Build history of the part. All positions in model axes, mm. Round coordinates to 2 decimals unless told otherwise and drop trailing zeros. Loops run counter-clockwise (first coordinate to the right, second up) from the corner with the lowest first, then second, coordinate; pieces in that order, holes last. Notation, with made-up numbers: (58.5, -1.75) - (77.5, -1.75) arc R13 ccw to (77.5, 7.25) - close; hole circle Ø4 at (79, 27.25). An arc over 180 degrees is marked (long way). Use a Markdown table: item, result.
from build123d import *

# Parameters (mm, degrees)
EXTRUDE_1_DEPTH        = 400
SKETCH_2_R             = 3
SKETCH_2_R_2           = 1.75
CUT_EXTRUDE_1_DEPTH    = 4.5
SKETCH_2_2_R           = 1.75
CUT_EXTRUDE_2_DEPTH    = 9
PATTERN_LINEAR_1_COUNT = 14
PATTERN_LINEAR_1_PITCH = 25
CROQUIS1_R             = 1.75
CORTAR_EXTRUIR1_DEPTH  = 8


with BuildPart() as part:
    # Эскиз1 → Бобышка-Вытянуть1 (new body)
    with BuildSketch(Plane.XY):
        with BuildLine():
            Line((-6, 3.7), (-5.7, 4))
            Line((-5.7, 4), (5.7, 4))
            Line((5.7, 4), (6, 3.7))
            Line((6, 3.7), (6, 2.451013544))
            ThreePointArc((6, 2.451013544), (5.597935912, 2.202976267), (5.354599002, 1.798050138))
            Line((5.354599002, 1.798050138), (4.643514056, 1.798050138))
            Line((4.643514056, 1.798050138), (4.643514056, 1.201949862))
            Line((4.643514056, 1.201949862), (5.354599002, 1.201949862))
            ThreePointArc((5.354599002, 1.201949862), (5.597935912, 0.797023733), (6, 0.548986456))
            Line((6, 0.548986456), (6, -3.7))
            Line((6, -3.7), (5.7, -4))
            Line((5.7, -4), (-5.7, -4))
            Line((-5.7, -4), (-6, -3.7))
            Line((-6, -3.7), (-6, 0.548986456))
            ThreePointArc((-6, 0.548986456), (-5.597935912, 0.797023733), (-5.354599002, 1.201949862))
            Line((-5.354599002, 1.201949862), (-4.643514056, 1.201949862))
            Line((-4.643514056, 1.201949862), (-4.643514056, 1.798050138))
            Line((-4.643514056, 1.798050138), (-5.354599002, 1.798050138))
            ThreePointArc((-5.354599002, 1.798050138), (-5.597935912, 2.202976267), (-6, 2.451013544))
            Line((-6, 2.451013544), (-6, 3.7))
        make_face()
    extrude(amount=EXTRUDE_1_DEPTH)

    # Эскиз2 → Вырез-Вытянуть1 (cut)
    with BuildSketch(Plane(origin=(0, 4, 0), x_dir=(1, 0, 0), z_dir=(0, 1, 0))):
        with Locations((0, -12)):
            Circle(SKETCH_2_R)
        with Locations((0, -12)):
            Circle(SKETCH_2_R_2, mode=Mode.SUBTRACT)
    cut_extrude_1 = extrude(amount=-CUT_EXTRUDE_1_DEPTH, mode=Mode.SUBTRACT)

    # Эскиз2<2> → Вырез-Вытянуть2 (cut, through all)
    with BuildSketch(Plane(origin=(0, 4, 0), x_dir=(1, 0, 0), z_dir=(0, 1, 0))):
        with Locations((0, -12)):
            Circle(SKETCH_2_2_R)
    cut_extrude_2 = extrude(amount=-CUT_EXTRUDE_2_DEPTH, mode=Mode.SUBTRACT)

    # Линейный массив1: Вырез-Вытянуть1, Вырез-Вытянуть2 ×14
    with Locations(*[(0, 0, i * PATTERN_LINEAR_1_PITCH) for i in range(1, PATTERN_LINEAR_1_COUNT)]):
        add(cut_extrude_1, mode=Mode.SUBTRACT)
        add(cut_extrude_2, mode=Mode.SUBTRACT)

    # Croquis1 → Cortar-Extruir1 (cut)
    with BuildSketch(Plane(origin=(0, 4, 0), x_dir=(1, 0, 0), z_dir=(0, 1, 0))):
        with Locations((0, -388)):
            Circle(CROQUIS1_R)
        with Locations((0, -363)):
            Circle(CROQUIS1_R)
    extrude(amount=-CORTAR_EXTRUIR1_DEPTH, mode=Mode.SUBTRACT)


solid = part.part
Q1. Drop flat-ended pins along their axis: pin 1 (5.5 mm diameter, centred on x = 0, z = 312, fed in from +Y); pin 2 (3 mm diameter, centred on x = 0, z = 37, fed in from +Y). Give the stop position or say it passes through.
Results found:
| item | result |
|---|---|
| pin 1 | stops at y = -0.5 |
| pin 2 | passes through |
Q2. Probe line 1 (Y direction, x = -5.25, z = 59.5); line 2 (X direction, y = -0.25, z = 137); line 3 (X direction, y = 1.75, z = 212). List the from-to ranges inside material, lowest first.
Results found:
| item | result |
|---|---|
| line 1 | y = -4 to 1.2, 1.8 to 4 |
| line 2 | x = -6 to -3, 3 to 6 |
| line 3 | x = -4.64 to -3, 3 to 4.64 |
Q3. Cut at A-A, the plane z = 245. List the corners of the cut face in (x, y), plus the area to 3 significant figures.
Results found:
| item | result |
|---|---|
| outline | (-6, -3.7) - (-5.7, -4) - (5.7, -4) - (6, -3.7) - (6, 0.55) arc R1 cw to (5.35, 1.2) - (4.64, 1.2) - (4.64, 1.8) - (5.35, 1.8) arc R1 cw to (6, 2.45) - (6, 3.7) - (5.7, 4) - (-5.7, 4) - (-6, 3.7) - (-6, 2.45) arc R1 cw to (-5.35, 1.8) - (-4.64, 1.8) - (-4.64, 1.2) - (-5.35, 1.2) arc R1 cw to (-6, 0.55) - close |
| area | 93.1 mm2 |
